from build123d import *

# Parameters (mm, degrees)
SKETCH1_R         = 4.0005
EXTRUDE1_DEPTH    = 2.921
FILLET1_R         = 1.524
SKETCH2_R         = 2.032
EXTRUDE2_DEPTH    = 12.065
SKETCH3_W         = 4.91456988
SKETCH3_H         = 0.615801824
EXTRUDE3_DEPTH    = 1.016
CIRPATTERN1_COUNT = 2
CIRPATTERN1_ANGLE = 90


with BuildPart() as part:
    # Sketch1 → Extrude1 (new body)
    with BuildSketch(Plane.XY):
        Circle(SKETCH1_R)
    extrude(amount=EXTRUDE1_DEPTH)

    # Fillet1
    fillet1_edges = [part.edges().sort_by_distance(p)[0] for p in [
        (-4.0005, 0, 0),
    ]]
    fillet(fillet1_edges, radius=FILLET1_R)

    # Sketch2 → Extrude2 (add)
    with BuildSketch(Plane.XY.offset(2.921)):
        Circle(SKETCH2_R)
    extrude(amount=EXTRUDE2_DEPTH)

    # Sketch3 → Extrude3 (cut)
    with BuildSketch(Plane(origin=(0, 0, 0), x_dir=(-1, 0, 0), z_dir=(0, 0, -1))):
        Rectangle(SKETCH3_W, SKETCH3_H)
    extrude3 = extrude(amount=-EXTRUDE3_DEPTH, mode=Mode.SUBTRACT)

    # CirPattern1: Extrude3 ×2 about axis
    cirpattern1_axis = Axis((0, 0, 0), (0, 0, -1))
    for i in range(1, CIRPATTERN1_COUNT):
        add(extrude3.rotate(cirpattern1_axis, i * CIRPATTERN1_ANGLE / (CIRPATTERN1_COUNT - 1)), mode=Mode.SUBTRACT)


solid = part.part
Can you work these out from the model? Positions are in its coordinate system, mm. A direction names the side the tool comes from. Coordinates: 2 decimals unless noted, no trailing zeros. Order: outer loops, then holes, each group sorted by start corner. A loop starts at its lowest first (then second) coordinate and runs counter-clockwise, first axis right, second up. Notation, with made-up numbers: M 71,-2.75 L 92,-2.75 A28 ccw 92,25.25 Z; hole C 71.5,70 d8. An arc over 180 degrees is marked long. Write item = value, one per line.
(1) If we mould it in two halves opening along Y, with no side actions, what happens to faces 4 (the face through (0, 0, 14.986)), 5 (the face through (-0.44, -1.984, 8.869)), 6 (the face through (0.308, -1.4, 0.5))? For each: pulls with the +Y half, pulls with the -Y half, needs draft (parallel to the pull), parting line crosses it, or undercut.
Results are:
face_4 = needs draft
face_5 = parting line crosses it
face_6 = undercut
(2) Suppose I cut it at C-C on z = 2.75. Please give me the cut outline in (x, y), plus the area to 3 significant figures.
Results are:
outline = C 0,0 d8
area = 50.3 mm2
(3) Suppose I cut it at D-D on z = 13. Please give me the cut outline in (x, y), plus the area to 3 significant figures.
Results are:
outline = C 0,0 d4.06
area = 13.0 mm2
(4) For pin 1 Ø1.5 at (x, y) = (-1, -1) entering from -Z; pin 2 Ø0.5 at (y, z) = (0, 0.5) entering from +X; pin 3 Ø1.5 at (x, z) = (2, 8.5) entering from -Y; pin 4 Ø0.5 at (x, z) = (-2, 1) entering from -Y, each with a flat end and sliding along its axis, tell me the tip position at first contact or that it passes through.
Results are:
pin_1 = 0
pin_2 = 3.79
pin_3 = -1.6
pin_4 = -3.52
(5) I need wall thicknesses on line 1 along Z through (x, y) = (1.25, 1.75); line 2 along Y through (x, z) = (0, 8.75); line 3 along Z through (x, y) = (0.25, -2.25). Which ranges of each line are inside material? Lowest first, please. Write a range as [from, to].
Results are:
line_1 = [0, 2.92]
line_2 = [-2.03, 2.03]
line_3 = [1.02, 2.92]
(6) For faces 1 (the face through (-1.4, -0.308, 0.5)), 2 (the face through (-2, 1, 2.921)), 3 (the face through (-0.9, -3.9, 2.2)), which set-ups out of +Z, -Z, +X, -X, +Y, -Y let a thin tool reach every point of the face, with its end or its side?
Results are:
face_1 = -Z
face_2 = +Z
face_3 = +Z, -Z
